```python
from build123d import *

# Parameters (mm, degrees)
SKETCH1_W           = 25
SKETCH1_H           = 24.7
SKETCH1_W_2         = 19
SKETCH1_H_2         = 18.5
BOSS_EXTRUDE1_DEPTH = 3.4
SKETCH1_3_W         = 33.6
SKETCH1_3_H         = 33.6
SKETCH1_3_W_2       = 25
SKETCH1_3_H_2       = 24.7
SKETCH1_3_W_3       = 19
SKETCH1_3_H_3       = 18.5
BOSS_EXTRUDE2_DEPTH = 27
SKETCH2_W           = 33.6
SKETCH2_H           = 33.6
BOSS_EXTRUDE3_DEPTH = 3
BOSS_EXTRUDE4_DEPTH = 6
FILLET1_R           = 5
SKETCH4_W           = 18
SKETCH4_H           = 5.2
CUT_EXTRUDE1_DEPTH  = 2.3
SKETCH5_W           = 17.2
SKETCH5_H           = 6.8
BOSS_EXTRUDE5_DEPTH = 1.1
SKETCH6_W           = 25
SKETCH6_H           = 6.2
CUT_EXTRUDE2_DEPTH  = 2.3
SKETCH7_W           = 1
SKETCH7_H           = 2.3
BOSS_EXTRUDE6_DEPTH = 6.2


with BuildPart() as part:
    # Sketch1 → Boss-Extrude1 (new body)
    with BuildSketch(Plane.XY):
        with Locations((0.492069479, 3.229581152)):
            Rectangle(SKETCH1_W, SKETCH1_H)
        with Locations((0.492069479, 5.329581152)):
            Rectangle(SKETCH1_W_2, SKETCH1_H_2, mode=Mode.SUBTRACT)
    extrude(amount=BOSS_EXTRUDE1_DEPTH)

    # Sketch1_3 → Boss-Extrude2 (add)
    # profile 1 of 2: a face of its own
    with BuildSketch(Plane.XY):
        with Locations((0.492069479, 0.879581152)):
            Rectangle(SKETCH1_3_W, SKETCH1_3_H)
        with Locations((0.492069479, 3.229581152)):
            Rectangle(SKETCH1_3_W_2, SKETCH1_3_H_2, mode=Mode.SUBTRACT)
    # profile 2 of 2: a face of its own
    with BuildSketch(Plane.XY):
        with Locations((0.492069479, 3.229581152)):
            Rectangle(SKETCH1_3_W_2, SKETCH1_3_H_2)
        with Locations((0.492069479, 5.329581152)):
            Rectangle(SKETCH1_3_W_3, SKETCH1_3_H_3, mode=Mode.SUBTRACT)
    extrude(amount=-BOSS_EXTRUDE2_DEPTH)

    # Sketch2 → Boss-Extrude3 (add)
    with BuildSketch(Plane(origin=(0, 0, -27), x_dir=(-1, 0, 0), z_dir=(0, 0, -1))):
        with Locations((-0.492069479, 0.879581152)):
            Rectangle(SKETCH2_W, SKETCH2_H)
    extrude(amount=BOSS_EXTRUDE3_DEPTH)

    # Sketch3 → Boss-Extrude4 (add)
    with BuildSketch(Plane(origin=(17.292069479, 0, 0), x_dir=(0, 0, -1), z_dir=(1, 0, 0))):
        with BuildLine():
            Line((2, -15.920418848), (2, -46.920418848))
            ThreePointArc((2, -46.920418848), (5.095135702, -38.140673143), (13.011990664, -33.242999493))
            ThreePointArc((13.011990664, -33.242999493), (12.948030778, -29.707093464), (16, -27.920418848))
            Line((16, -27.920418848), (16, -15.920418848))
            Line((16, -15.920418848), (2, -15.920418848))
        make_face()
        with BuildLine():
            ThreePointArc((18.988009336, -33.242999493), (26.904864298, -38.140673143), (30, -46.920418848))
            Line((30, -46.920418848), (30, -15.920418848))
            Line((30, -15.920418848), (16, -15.920418848))
            Line((16, -15.920418848), (16, -27.920418848))
            ThreePointArc((16, -27.920418848), (18.474873734, -28.945545114), (19.5, -31.420418848))
            ThreePointArc((19.5, -31.420418848), (19.36957213, -32.366982983), (18.988009336, -33.242999493))
        make_face()
        with BuildLine():
            ThreePointArc((16, -43.420418848), (18.474873734, -44.445545114), (19.5, -46.920418848))
            Line((19.5, -46.920418848), (30, -46.920418848))
            ThreePointArc((30, -46.920418848), (26.904864298, -38.140673143), (18.988009336, -33.242999493))
            ThreePointArc((18.988009336, -33.242999493), (17.713325384, -34.47238807), (16, -34.920418848))
            Line((16, -34.920418848), (16, -43.420418848))
        make_face()
        with BuildLine():
            Line((2, -46.920418848), (12.5, -46.920418848))
            ThreePointArc((12.5, -46.920418848), (13.525126266, -44.445545114), (16, -43.420418848))
            Line((16, -43.420418848), (16, -34.920418848))
            ThreePointArc((16, -34.920418848), (14.286674616, -34.47238807), (13.011990664, -33.242999493))
            ThreePointArc((13.011990664, -33.242999493), (5.095135702, -38.140673143), (2, -46.920418848))
        make_face()
        with BuildLine():
            Line((30, -46.920418848), (19.5, -46.920418848))
            ThreePointArc((19.5, -46.920418848), (16, -50.420418848), (12.5, -46.920418848))
            Line((12.5, -46.920418848), (2, -46.920418848))
            ThreePointArc((2, -46.920418848), (16, -60.920418848), (30, -46.920418848))
        make_face()
    extrude(amount=-BOSS_EXTRUDE4_DEPTH)

    # Fillet1
    fillet1_edges = [part.edges().sort_by_distance(p)[0] for p in [
        (17.292069479, 17.679581152, -15),
        (-16.307930521, -15.920418848, -15),
        (-16.307930521, 17.679581152, -15),
        (17.292069479, -15.920418848, -1),
    ]]
    fillet(fillet1_edges, radius=FILLET1_R)

    # Sketch4 → Cut-Extrude1 (cut)
    with BuildSketch(Plane.XY.offset(3.4)):
        with Locations((0.492069479, -6.520418848)):
            Rectangle(SKETCH4_W, SKETCH4_H)
    extrude(amount=-CUT_EXTRUDE1_DEPTH, mode=Mode.SUBTRACT)

    # Sketch5 → Boss-Extrude5 (add)
    with BuildSketch(Plane.XY):
        with Locations((0.492069479, -12.520418848)):
            Rectangle(SKETCH5_W, SKETCH5_H)
    extrude(amount=BOSS_EXTRUDE5_DEPTH)

    # Sketch6 → Cut-Extrude2 (cut)
    with BuildSketch(Plane.XY.offset(3.4)):
        with Locations((0.492069479, -6.020418848)):
            Rectangle(SKETCH6_W, SKETCH6_H)
    extrude(amount=-CUT_EXTRUDE2_DEPTH, mode=Mode.SUBTRACT)

    # Sketch7 → Boss-Extrude6 (add)
    with BuildSketch(Plane.XZ.offset(2.920418848)):
        with Locations((-11.507930521, 2.25)):
            Rectangle(SKETCH7_W, SKETCH7_H)
        with Locations((12.492069479, 2.25)):
            Rectangle(SKETCH7_W, SKETCH7_H)
    extrude(amount=BOSS_EXTRUDE6_DEPTH)


solid = part.part
```
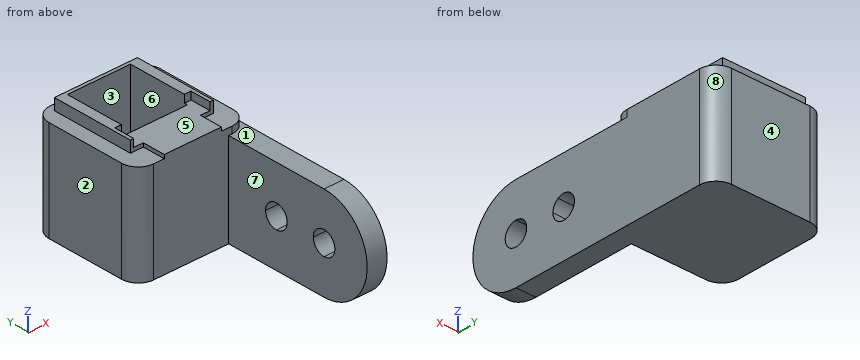
Work out the finished part from the listing and answer in its coordinate system (mm). Face numbers are marked on the shaded views. A direction names the side the tool comes from. Round coordinates to 2 decimals unless told otherwise and drop trailing zeros. Write each loop counter-clockwise with the first axis right and the second up, starting at its lowest first coordinate (ties: lowest second). Pieces come first, ordered by that corner, then holes. Notation, with made-up numbers: (23, 23.25) -> (55, 23.25) arc R21 ccw to (55, 59.25) -> close; hole circle Ø5 at (45.25, 56). An arc over 180 degrees is marked (long way). Write each question's results on one line, items separated by ' | '.
1) Flat-ended cylindrical pins translate along their axes: pin 1 (1.7 mm diameter, centred on y = 0.5, z = 1.5, fed in from -X); pin 2 (1.2 mm diameter, centred on y = -14, z = 0.5, fed in from -X); pin 3 (6.5 mm diameter, centred on x = 13.5, y = -25, fed in from +Z); pin 4 (17 mm diameter, centred on x = -3, y = -6, fed in from +Z). Find the tip coordinate at first contact, or state that the pin passes through.
Findings:
pin 1: stops at x = -12.01 | pin 2: stops at x = -15.49 | pin 3: stops at z = -2 | pin 4: stops at z = 3.4
2) The part is cut by section A-A (z = -17.5). Write down the section's boundary in (x, y).
Findings:
outline: (-16.31, -10.92) arc R5 ccw to (-11.31, -15.92) -> (11.29, -15.92) -> (11.29, -28.26) -> (17.29, -28.26) -> (17.29, 12.68) arc R5 ccw to (12.29, 17.68) -> (-11.31, 17.68) arc R5 ccw to (-16.31, 12.68) -> close; (11.29, -60.84) -> (17.29, -60.84) -> (17.29, -50.08) -> (11.29, -50.08) -> close; (11.29, -43.76) -> (17.29, -43.76) -> (17.29, -34.58) -> (11.29, -34.58) -> close; hole (-9.01, -3.92) -> (9.99, -3.92) -> (9.99, 14.58) -> (-9.01, 14.58) -> close
3) The part is cut by section B-B (y = -6.5). Write down the section's boundary in (x, z), and give its area (3 significant figures).
Findings:
outline: (-16.31, -30) -> (17.29, -30) -> (17.29, 0) -> (12.99, 0) -> (12.99, 3.4) -> (11.99, 3.4) -> (11.99, 1.1) -> (-11.01, 1.1) -> (-11.01, 3.4) -> (-12.01, 3.4) -> (-12.01, 0) -> (-16.31, 0) -> close | area: 1,040 mm²
4) For a pull along X with two mould halves and no side action, classify the marked faces 1, 2 and 3 as +X half, -X half, draft (parallel to the pull), parting line (faces both ways), or undercut.
Findings:
face 1: draft | face 2: -X half | face 3: undercut
5) Which of the six approach directions +Z, -Z, +X, -X, +Y, -Y give full straight-line access (tool end or side, diameter ignored) to the marked faces 4, 5, 6, 7 and 8?
Findings:
face 4: +Z, -Z, +X, -X, +Y | face 5: +Z, -Y | face 6: +Z | face 7: +Z, -Z, -X, -Y | face 8: +Z, -Z, +X, +Y
6) The part is cut by section D-D (y = -18). Write down the section's boundary in (x, z).
Findings:
outline: (11.29, -30) -> (17.29, -30) -> (17.29, -2) -> (11.29, -2) -> close
7) The part is cut by section C-C (x = -1.5). Write down the section's boundary in (y, z).
Findings:
outline: (-15.92, -30) -> (17.68, -30) -> (17.68, 0) -> (15.58, 0) -> (15.58, 3.4) -> (14.58, 3.4) -> (14.58, -27) -> (-3.92, -27) -> (-3.92, 1.1) -> (-15.92, 1.1) -> close
8) Consider line 1 along X through (y, z) = (8.5, -9.5); line 2 along Y through (x, z) = (9.5, -25.5); line 3 along Y through (x, z) = (15, -13). Determine where each line is inside the solid, lowest interval first. Write a range as [from, to].
Findings:
line 1: x = [-16.31, -9.01], [9.99, 17.29] | line 2: y = [-15.92, -3.92], [14.58, 17.68] | line 3: y = [-60.6, -48.72], [-45.12, -33.22], [-29.62, 16.88]
